Design review of the part shown in the three views and the two pictorial views. Dimensions are in mm from the part's minimum x, y and z. Give positions to 0.01 mm unless a question says otherwise; leave off trailing zeros. Order: outer loops, then holes, each group sorted by start corner. A loop starts at its lowest first (then second) coordinate and runs counter-clockwise, first axis right, second up. Notation, with made-up numbers: M 33,83.5 L 37,83.5 A17 ccw 37,114.5 Z; hole C 89.25,-33.75 d1. An arc over 180 degrees is marked long. Answer as a JSON object with one key per item and string values.
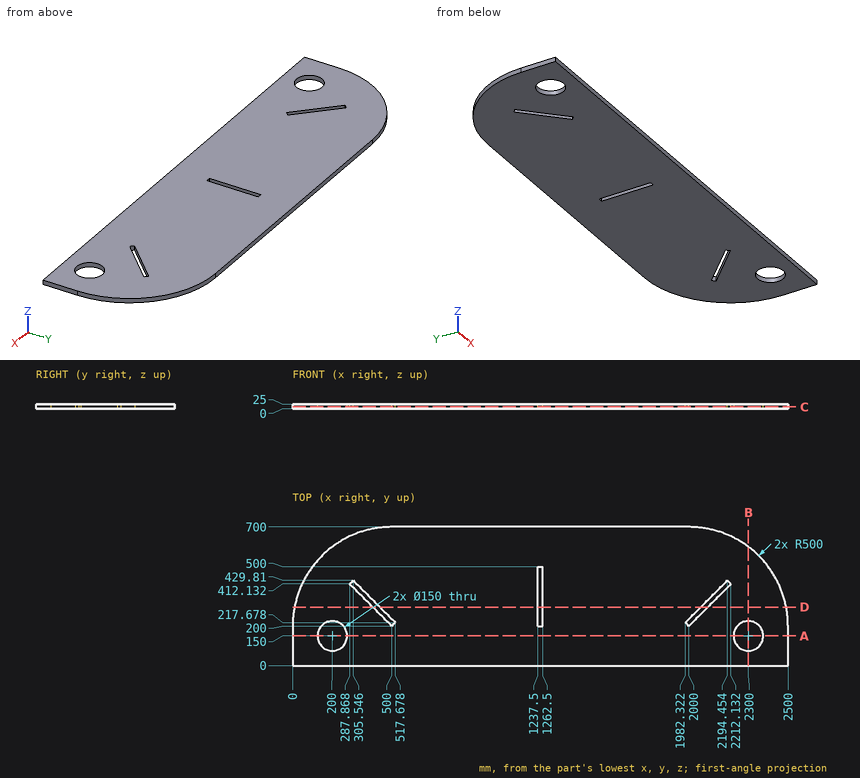
(1) We need section B-B (x = 2300). Write out the cut boundary in (y, z), plus the area to 4 significant figures.
Checked values:
{"outline": "M 0,0 L 75,0 L 75,25 L 0,25 Z; M 225,0 L 600,0 L 600,25 L 225,25 Z", "area": "11,250 mm^2"}
(2) To check wall thickness, follow L1, parallel to X at y = 97, z = 4 (1 decimal); L2, parallel to X at y = 411.5, z = 7.75 (1 decimal); L3, parallel to Y at x = 2360.5, z = 8.25 (1 decimal). State the ranges of each line that lie inside material, in increasing order. Write a range as from..to.
Checked values:
{"L1": "x = 0..146.9, 253.1..2246.9, 2353.1..2500", "L2": "x = 46.9..288.5, 323.9..1237.5, 1262.5..2176.1, 2211.5..2453.1", "L3": "y = 0..105.7, 194.3..546.5"}
(3) We need section A-A (y = 150). Write out the cut boundary in (x, z).
Checked values:
{"outline": "M 0,0 L 125,0 L 125,25 L 0,25 Z; M 275,0 L 2225,0 L 2225,25 L 275,25 Z; M 2375,0 L 2500,0 L 2500,25 L 2375,25 Z"}
(4) Insertion check: pin 1 (7.5 mm diameter, centred on x = 1251, z = 17, fed in from -Y); pin 2 (7.5 mm diameter, centred on y = 334, z = 10.5, fed in from -X); pin 3 (7.5 mm diameter, centred on y = 405, z = 15, fed in from +X); pin 4 (5 mm diameter, centred on y = 532.5, z = 22.5, fed in from +X). Each pin has a flat end and moves straight along its axis. Give the tip position at first contact, or say it passes through.
Checked values:
{"pin 1": "stops at y = 0", "pin 2": "stops at x = 17.26", "pin 3": "stops at x = 2457.71", "pin 4": "stops at x = 2375.63"}
(5) We need section D-D (y = 295). Write out the cut boundary in (x, z) (1 decimal).
Checked values:
{"outline": "M 9.1,0 L 405,0 L 405,25 L 9.1,25 Z; M 440.4,0 L 1237.5,0 L 1237.5,25 L 440.4,25 Z; M 1262.5,0 L 2059.6,0 L 2059.6,25 L 1262.5,25 Z; M 2095,0 L 2490.9,0 L 2490.9,25 L 2095,25 Z"}
(6) We need section C-C (z = 10). Write out the cut boundary in (x, y) (1 decimal).
Checked values:
{"outline": "M 0,0 L 2500,0 L 2500,200 A500 ccw 2000,700 L 500,700 A500 ccw 0,200 Z; hole C 200,150 d150; hole M 287.9,412.1 L 500,200 L 517.7,217.7 L 305.5,429.8 Z; hole M 1237.5,200 L 1262.5,200 L 1262.5,500 L 1237.5,500 Z; hole M 1982.3,217.7 L 2000,200 L 2212.1,412.1 L 2194.5,429.8 Z; hole C 2300,150 d150"}
